```python
from build123d import *

# Parameters (mm, degrees)
SKETCH1_W                = 20
SKETCH1_H                = 42
SKETCH1_W_2              = 42
BOSS_EXTRUDE1_DEPTH      = 6
SKETCH2_R                = 11.25
CUT_EXTRUDE1_DEPTH       = 3
CUT_EXTRUDE2_DEPTH       = 47.454278597
CUT_EXTRUDE2_DEPTH_BACK  = 47.454278597
SKETCH3_R                = 1.75
SKETCH3_R_2              = 6
CUT_EXTRUDE3_START       = -3
SKETCH4_R                = 3
SKETCH4_R_2              = 1.75
CUT_EXTRUDE3_DEPTH       = 3
SKETCH5_W                = 4.5
SKETCH5_H                = 42
BOSS_EXTRUDE2_DEPTH      = 3
CHAMFER1_SIZE            = 3
CUT_EXTRUDE4_DEPTH       = 47.936126811
CUT_EXTRUDE4_DEPTH_BACK  = 47.936126811
SKETCH6_R                = 2.75
SKETCH7_W                = 9.456435582
SKETCH7_H                = 20
SKETCH7_R                = 2.75
CUT_EXTRUDE5_DEPTH       = 47.454278597
BOSS_EXTRUDE4_DEPTH      = 3
BOSS_EXTRUDE4_DEPTH_BACK = 6
SKETCH8_W                = 20
SKETCH8_H                = 42
SKETCH8_R                = 7
CHAMFER2_SIZE            = 4
SKETCH9_R                = 50
CUT_EXTRUDE7_DEPTH       = 1.5
CUT_EXTRUDE8_START       = -1.5
SKETCH10_R               = 3
CUT_EXTRUDE8_DEPTH       = 1.5


with BuildPart() as part:
    # Sketch1 → Boss-Extrude1 (new body)
    with BuildSketch(Plane.XY):
        with Locations((31, 0)):
            Rectangle(SKETCH1_W, SKETCH1_H)
        Rectangle(SKETCH1_W_2, SKETCH1_H)
    extrude(amount=BOSS_EXTRUDE1_DEPTH)

    # Sketch2 → Cut-Extrude1 (cut)
    with BuildSketch(Plane.XY):
        Circle(SKETCH2_R)
    extrude(amount=CUT_EXTRUDE1_DEPTH, mode=Mode.SUBTRACT)

    # Sketch3 → Cut-Extrude2 (cut, two sides: drawn at the far end of the back side and taken through both)
    with BuildSketch(Plane.XY.offset(-CUT_EXTRUDE2_DEPTH_BACK)):
        with Locations((-15.499780644, 15.499780644)):
            Circle(SKETCH3_R)
        Circle(SKETCH3_R_2)
        with Locations((15.499780644, 15.499780644)):
            Circle(SKETCH3_R)
        with Locations((15.499780644, -15.499780644)):
            Circle(SKETCH3_R)
        with Locations((-15.499780644, -15.499780644)):
            Circle(SKETCH3_R)
    extrude(amount=CUT_EXTRUDE2_DEPTH + CUT_EXTRUDE2_DEPTH_BACK, mode=Mode.SUBTRACT)

    # Sketch4 → Cut-Extrude3 (cut)
    # profile 1 of 4: a face of its own
    with BuildSketch(Plane.XY.offset(6).offset(CUT_EXTRUDE3_START)):
        with Locations((-15.499780644, -15.499780644)):
            Circle(SKETCH4_R)
        with Locations((-15.499780644, -15.499780644)):
            Circle(SKETCH4_R_2, mode=Mode.SUBTRACT)
    # profile 2 of 4: a face of its own
    with BuildSketch(Plane.XY.offset(6).offset(CUT_EXTRUDE3_START)):
        with Locations((-15.499780644, 15.499780644)):
            Circle(SKETCH4_R)
        with Locations((-15.499780644, 15.499780644)):
            Circle(SKETCH4_R_2, mode=Mode.SUBTRACT)
    # profile 3 of 4: a face of its own
    with BuildSketch(Plane.XY.offset(6).offset(CUT_EXTRUDE3_START)):
        with Locations((15.499780644, 15.499780644)):
            Circle(SKETCH4_R)
        with Locations((15.499780644, 15.499780644)):
            Circle(SKETCH4_R_2, mode=Mode.SUBTRACT)
    # profile 4 of 4: a face of its own
    with BuildSketch(Plane.XY.offset(6).offset(CUT_EXTRUDE3_START)):
        with Locations((15.499780644, -15.499780644)):
            Circle(SKETCH4_R)
        with Locations((15.499780644, -15.499780644)):
            Circle(SKETCH4_R_2, mode=Mode.SUBTRACT)
    extrude(amount=CUT_EXTRUDE3_DEPTH, mode=Mode.SUBTRACT)

    # Sketch5 → Boss-Extrude2 (add)
    with BuildSketch(Plane.XY.offset(6)):
        with Locations((31, 0)):
            Rectangle(SKETCH5_W, SKETCH5_H)
    extrude(amount=BOSS_EXTRUDE2_DEPTH)

    # Chamfer1
    chamfer1_edges = [part.edges().sort_by_distance(p)[0] for p in [
        (-21, -21, 3),
        (-21, 21, 3),
    ]]
    chamfer(chamfer1_edges, length=CHAMFER1_SIZE)

    # Sketch6 → Cut-Extrude4 (cut, two sides: drawn at the far end of the back side and taken through both)
    with BuildSketch(Plane(origin=(0, 0, 0), x_dir=(-1, 0, 0), z_dir=(0, 0, -1)).offset(-CUT_EXTRUDE4_DEPTH_BACK)):
        with Locations(Location((-31, 0, 0), (0, 0, 324.903198772))):
            Circle(SKETCH6_R)
    extrude(amount=CUT_EXTRUDE4_DEPTH + CUT_EXTRUDE4_DEPTH_BACK, mode=Mode.SUBTRACT)

    # Sketch7 → Cut-Extrude5 (cut, through all)
    with BuildSketch(Plane.XY.offset(6)):
        with Locations((31, 0)):
            Rectangle(SKETCH7_W, SKETCH7_H)
        with Locations((31, 0)):
            Circle(SKETCH7_R, mode=Mode.SUBTRACT)
    extrude(amount=CUT_EXTRUDE5_DEPTH, mode=Mode.SUBTRACT)

    # Sketch8 → Boss-Extrude4 (add, two sides: drawn at the far end of the back side and taken through both)
    # profile 1 of 2: a face of its own
    with BuildSketch(Plane(origin=(0, 0, 0), x_dir=(-1, 0, 0), z_dir=(0, 0, -1)).offset(-BOSS_EXTRUDE4_DEPTH_BACK)):
        Polygon((18, -21), (-21, -21), (-41, -21), (-41, -24), (24, -24), (24, 24), (-41, 24), (-41, 21), (-21, 21), (18, 21), (21, 18), (21, -18), align=None)
    # profile 2 of 2: a face of its own
    with BuildSketch(Plane(origin=(0, 0, 0), x_dir=(-1, 0, 0), z_dir=(0, 0, -1)).offset(-BOSS_EXTRUDE4_DEPTH_BACK)):
        with Locations((-31, 0)):
            Rectangle(SKETCH8_W, SKETCH8_H)
        with Locations((-31, 0)):
            Circle(SKETCH8_R, mode=Mode.SUBTRACT)
    extrude(amount=BOSS_EXTRUDE4_DEPTH + BOSS_EXTRUDE4_DEPTH_BACK)

    # Chamfer2
    chamfer2_edges = [part.edges().sort_by_distance(p)[0] for p in [
        (-24, 24, 1.5),
        (-24, -24, 1.5),
    ]]
    chamfer(chamfer2_edges, length=CHAMFER2_SIZE)

    # Sketch9 → Cut-Extrude7 (cut)
    with BuildSketch(Plane.XY.offset(6)):
        with Locations((-40, 0)):
            Circle(SKETCH9_R)
    extrude(amount=-CUT_EXTRUDE7_DEPTH, mode=Mode.SUBTRACT)

    # Sketch10 → Cut-Extrude8 (cut)
    with BuildSketch(Plane.XY.offset(3).offset(CUT_EXTRUDE8_START)):
        with Locations((-15.499780644, 15.499780644)):
            Circle(SKETCH10_R)
        with Locations((-15.499780644, -15.499780644)):
            Circle(SKETCH10_R)
    extrude(amount=CUT_EXTRUDE8_DEPTH, mode=Mode.SUBTRACT)


solid = part.part
```
CAD build for the part. Positions are in the model's coordinates, mm. A direction names the side the tool comes from. Coordinates: 2 decimals unless noted, no trailing zeros. Loops run counter-clockwise (first coordinate to the right, second up) from the corner with the lowest first, then second, coordinate; pieces in that order, holes last. Notation, with made-up numbers: (11.5, 66) - (64.5, 66) arc R22 cw to (64.5, 82) - close; hole circle Ø9 at (-27, 83.25). An arc over 180 degrees is marked (long way). Return JSON: item names as keys, results as strings.
1. Band-saw the part on D-D (z = -1). Give the cut face in (x, y), and give its area (3 significant figures).
Result:
{"outline": "(-24, -20) - (-20, -24) - (41, -24) - (41, 24) - (-20, 24) - (-24, 20) - close; hole (-21, -18) - (-18, -21) - (21, -21) - (21, 21) - (-18, 21) - (-21, 18) - close; hole circle Ø14 at (31, 0)", "area": "1,200 mm2"}
2. Mould opens along Y. For faces 1 (the flat face through (9, -9, 0)), 2 (the flat face through (31, -21, 7)), 3 (the flat face through (31, 21, 7)) say: released by +Y, released by -Y, zero draft, split by the parting line, or undercut.
Result:
{"face 1": "undercut", "face 2": "released by -Y", "face 3": "released by +Y"}
3. Probe L1, parallel to Y at x = 0, z = 2.05; L2, parallel to Z at x = 37, y = 20.5; L3, parallel to Z at x = 17, y = -19. List the from-to ranges inside material, lowest first. Write a range as from..to.
Result:
{"L1": "y = -24..-11.25, 11.25..24", "L2": "z = -3..6", "L3": "z = 0..6"}
4. Band-saw the part on C-C (y = 0). Give the cut face in (x, z), and give its area (4 significant figures).
Result:
{"outline": "(-24, -3) - (-21, -3) - (-21, 0) - (-11.25, 0) - (-11.25, 3) - (-6, 3) - (-6, 4.5) - (-24, 4.5) - close; (6, 3) - (11.25, 3) - (11.25, 0) - (21, 0) - (21, -3) - (24, -3) - (24, 0) - (28.25, 0) - (28.25, 6) - (10, 6) - (10, 4.5) - (6, 4.5) - close; (33.75, 0) - (38, 0) - (38, -3) - (41, -3) - (41, 6) - (33.75, 6) - close", "area": "247.5 mm2"}
5. Band-saw the part on A-A (x = 31). Give the cut face in (y, z), and give its area (3 significant figures).
Result:
{"outline": "(-24, -3) - (-7, -3) - (-7, 0) - (-2.75, 0) - (-2.75, 6) - (-10, 6) - (-10, 9) - (-21, 9) - (-21, 6) - (-24, 6) - close; (2.75, 0) - (7, 0) - (7, -3) - (24, -3) - (24, 6) - (21, 6) - (21, 9) - (10, 9) - (10, 6) - (2.75, 6) - close", "area": "423 mm2"}
6. Band-saw the part on B-B (z = 7.25). Give the cut face in (x, y).
Result:
{"outline": "(28.75, -21) - (33.25, -21) - (33.25, -10) - (28.75, -10) - close; (28.75, 10) - (33.25, 10) - (33.25, 21) - (28.75, 21) - close"}
7. 3-axis set-ups, long thin cutter, end or side, ignore diameter. For faces 4 (the flat face through (33.25, -16, 7)), 5 (the cylindrical face through (10, 0, 5)), 6 (the cylindrical face through (12.5, -15.4, 4.5)), 7 (the flat face through (31, 16, 9)), 8 (the flat face through (-21, 0, -1)): which of +Z, -Z, +X, -X, +Y, -Y reach the whole face in a straight line?
Result:
{"face 4": "+Z, +X, +Y, -Y", "face 5": "+Z, -X", "face 6": "+Z", "face 7": "+Z, +X, -X, +Y, -Y", "face 8": "-Z"}
8. Drop flat-ended pins along their axis: pin 1 (1 mm diameter, centred on x = -5, y = -10.5, fed in from -Z); pin 2 (11 mm diameter, centred on x = 13.5, y = -11, fed in from +Z); pin 3 (3 mm diameter, centred on x = -14.5, y = 15, fed in from +Z). Give the stop position or say it passes through.
Result:
{"pin 1": "stops at z = 0", "pin 2": "stops at z = 6", "pin 3": "stops at z = 1.5"}
